Can you work these out from the model? Positions are in its coordinate system, mm. A direction names the side the tool comes from. Round coordinates to 2 decimals unless told otherwise and drop trailing zeros. Loops run counter-clockwise (first coordinate to the right, second up) from the corner with the lowest first, then second, coordinate; pieces in that order, holes last. Notation, with made-up numbers: (70, -19.5) -> (103, -19.5) arc R27 cw to (103, 8.5) -> close; hole circle Ø6 at (-5, 1.5). An arc over 180 degrees is marked (long way). Use a Markdown table: item, result.
Autodesk Inventor part; units mm, degrees
ref_plane "Work Plane1" through (29, 0, 0) normal (0, -1, 0) x (1, 0, 0)
ref_plane "YZ Plane" through (0, 0, 0) normal (1, 0, 0) x (0, 1, 0)
ref_plane "XZ Plane" through (0, 0, 0) normal (0, 1, 0) x (-1, 0, 0)
sketch "Skizze1" plane through (0, 0, 0) normal (0, 0, 1) x (1, 0, 0)
  line L0 (-1, 0) -> (20, 0)
  line L1 (20, 0) -> (20, 2)
  line L2 (20, 2) -> (1.75, 2)
  line L3 (1.75, 2) -> (1.3205, 2)
  line L4 (1.3205, 2) -> (0, 2)
  line L5 (0, 2) -> (0, 3.5)
  line L6 (0, 3.5) -> (-4, 3.5)
  line L7 (-4, 3.5) -> (-4, 1.7321)
  line L8 (-4, 1.7321) -> (-2, 1.7321)
  line L9 (-2, 1.7321) -> (-1, 0)
  line L10 (-8.8, 0) -> (24.8, 0)
  line L11 (0, -0.7) -> (0, 4.2)
  line L12 (1.75, 2) -> (0, 2) construction
  dimension "d1" = 18.25
  dimension "d2" = 0.4295
  dimension "d3" = 4
  dimension "d4" = 2
  dimension "d5" = 60
  dimension "d6" = 4
  dimension "d7" = 4
  dimension "d8" = 3.4641
  dimension "d9" = 7
  dimension "d26" = 20
revolve "Körper" add sketch "Skizze1" angle 360 about axis through (-1, 0, 0) along (1, 0, 0)
sketch "Skizze2" plane through (-4, 0, 0) normal (-1, 0, 0) x (0, 0, 1)
  circle A0 centre (0, 0) radius 1.7321
  line L0 (0, -4.9) -> (0, 4.9)
  line L1 (-4.9, 0) -> (4.9, 0)
  line L2 (1.7321, 0) -> (0.866, -1.5)
  line L3 (0.866, -1.5) -> (-0.866, -1.5)
  line L4 (-0.866, -1.5) -> (-1.7321, 0)
  line L5 (-1.7321, 0) -> (-0.866, 1.5)
  line L6 (-0.866, 1.5) -> (0.866, 1.5)
  line L7 (0.866, 1.5) -> (1.7321, 0)
extrude "Loch" add sketch "Skizze2" against normal up to next contours L7 A0 | A0 L2 | L6 L0 A0 | A0 L0 L3 | L0 L6 A0 | A0 L3 L0 | L4 A0 | A0 L5
fillet "Rundung1" radius 0.4 1 edges at (-4, -3.5, 0)
thread "Gewinde"
chamfer "Fase1" distance 0.4294 distance2 0.4294 1 edges at (20, -2, 0) measured on face at (20, 0.0679, 1.2634)
ref_plane "Work Plane1" through (29, 0, 0) normal (0, -1, 0) x (1, 0, 0)
fillet "Fillet2" radius 0.1 1 edges at (0, -2, 0)
sketch "Skizze4" plane through (0, 0, 0) normal (0, 1, 0) x (-1, 0, 0)
  line L0 (8.8, 0) -> (-24.8, 0)
  line L1 (-5, 2) -> (-5.64, 2)
  line L2 (-5.64, 2) -> (-5.64, 1.15)
  line L3 (-5.64, 1.15) -> (-5, 1.15)
  line L4 (-5, 1.15) -> (-5, 2)
  line L5 (-0.1, 2) -> (-19.5706, 2)
  line L6 (0, 3.5) -> (0, -3.5)
  line L7 (3.6, -3.5) -> (3.6, 3.5)
  point P0 (0, 0)
  dimension "d31" = 5
  dimension "d32" = 0.64
  dimension "d33" = 2.3
revolve "Umdrehung2" cut sketch "Skizze4" angle 360 about axis through (-10, 0, 0) along (1, 0, 0)
equation "\"d30\" = R"
equation "\"d17\" = RR"
equation "\"d13\" = GEL"
equation "\"d15\" = -0.5 * SPD + 0.5 * GD"
equation "\"d16\" = GUL"
equation "\"d1\" = GEL"
equation "\"d3\" = KOH"
equation "\"d4\" = INTI"
equation "\"d6\" = GD"
equation "\"d7\" = BDM"
equation "\"d8\" = 1.1547 * SW"
equation "\"d9\" = KOD"
equation "\"d26\" = NLG"
equation "\"GD\" = 4"
equation "\"NLG\" = 20"
equation "\"GEL\" = 18.25"
equation "\"KOD\" = 7"
equation "\"KOH\" = 4"
equation "\"INTI\" = 2"
equation "\"GAL\" = 0.61345 * PTC"
equation "\"GUL\" = 0.61345 * PTC"
equation "\"BDM\" = NND"
equation "\"SW\" = 3"
equation "\"RR\" = 0.4"
equation "\"SPD\" = NND - 1.2269 * PTC"
equation "\"R\" = 0.1"
equation "\"TOA\" = 30deg"
equation "\"GD1\" = THREADDIA - 1.2269 * PTC"
equation "\"THREADDIA\" = 4"
equation "\"FAWI\" = 45deg"
equation "\"PTC\" = 0.7"
equation "\"NND\" = 4"
equation "\"E0\" = 1.155 * SW"
properties part number "ISO 4762 - M4 x 20" material "EdelStahl - 440C"
1. If we mould it in two halves opening along Y, with no side actions, what happens to faces 1 (the flat face through (-2.948, 0.74, -1.305)), 2 (the flat face through (5, 1, 1)), 3 (the cylindrical face through (-1.825, 3.233, 1.341))? For each: +Y half, -Y half, draft (parallel to the pull), parting line (faces both ways), or undercut.
Answer sheet:
| item | result |
|---|---|
| face 1 | undercut |
| face 2 | draft |
| face 3 | parting line |
2. I want a section at A-A (x = 0.5). Please give me the cut outline in (y, z).
Answer sheet:
| item | result |
|---|---|
| outline | circle Ø4 at (0, 0) |
3. Which directions (+Z, -Z, +X, -X, +Y, -Y) give clear straight access to the entire face, cutting with the end or side of a thin tool? Please do faces 4 (the flat face through (5.64, 1, 1)), 5 (the flat face through (-2.948, 0.761, 1.293)), 6 (the cylindrical face through (3, 0, 2)).
Answer sheet:
| item | result |
|---|---|
| face 4 | none |
| face 5 | -X |
| face 6 | +X |
4. Will these pins go through, and if not, where does the flat tip stop? pin 1 Ø1.5 at (x, y) = (8.5, 2) entering from +Z; pin 2 Ø1.2 at (y, z) = (0.5, 0) entering from -X; pin 3 Ø4 at (x, z) = (14.5, -2.5) entering from +Y.
Answer sheet:
| item | result |
|---|---|
| pin 1 | stops at z = 1.56 |
| pin 2 | stops at x = -1.64 |
| pin 3 | stops at y = 1.94 |
5. I need wall thicknesses on line 1 (X direction, y = 0.25, z = -1.25); line 2 (Y direction, x = 7.75, z = -1); line 3 (X direction, y = 0, z = 1.5). Which ranges of each line are inside material? Lowest first, please.
Answer sheet:
| item | result |
|---|---|
| line 1 | x = -1.74 to 5, 5.64 to 20 |
| line 2 | y = -1.73 to 1.73 |
| line 3 | x = -1.87 to 5, 5.64 to 20 |
